Autodesk Inventor part; units mm, degrees
ref_plane "Work Plane1" through (104.775, 0, 0) normal (0, 0, -1) x (1, 0, 0)
ref_plane "YZ Plane" through (0, 0, 0) normal (1, 0, 0) x (0, 1, 0)
ref_plane "XZ Plane" through (0, 0, 0) normal (0, 1, 0) x (-1, 0, 0)
sketch "Esquisse1" plane through (0, 0, 0) normal (0, 0, 1) x (1, 0, 0)
  line L0 (16, 0) -> (16, 2)
  line L1 (16, 2) -> (4.6, 2)
  line L2 (4.6, 2) -> (4.1706, 2)
  line L3 (0, 4) -> (0, 1.4434)
  line L4 (0, 1.4434) -> (1.49, 1.4434)
  line L5 (1.49, 1.4434) -> (2.3233, 0)
  line L6 (2.3233, 0) -> (16, 0)
  line L7 (0, 4) -> (0.48, 4)
  line L8 (0.48, 4) -> (2.48, 2)
  line L9 (4.1706, 2) -> (2.48, 2)
  line L10 (4.6, 2) -> (2.48, 2) construction
  line L11 (2.48, 2) -> (2.48, 2)
  line L12 (-3.2, 0) -> (19.2, 0)
  line L13 (0, -0.8) -> (0, 4.8)
  dimension "d0" = 16
  dimension "d1" = 11.4
  dimension "d2" = 1.49
  dimension "d3" = 4
  dimension "d6" = 2.48
  dimension "d7" = 45
  dimension "d8" = 2.8868
  dimension "d9" = 60
  dimension "d10" = 8
  dimension "d11" = 4
  dimension "d12" = 0.4294
revolve "Corps" add sketch "Esquisse1" angle 360 about axis through (2.3233, 0, 0) along (1, 0, 0) contours L6 L5 L4 L3 L7 L8 L9 L2 L1 L0
sketch "Esquisse2" plane through (0, 0, 0) normal (-1, 0, 0) x (0, 0, 1)
  circle A0 centre (0, 0) radius 1.4434
  line L0 (0, -5.6) -> (0, 5.6)
  line L1 (-5.6, 0) -> (5.6, 0)
  line L2 (1.4434, 0) -> (0.7217, -1.25)
  line L3 (0.7217, -1.25) -> (-0.7217, -1.25)
  line L4 (-0.7217, -1.25) -> (-1.4434, 0)
  line L5 (-1.4434, 0) -> (-0.7217, 1.25)
  line L6 (-0.7217, 1.25) -> (0.7217, 1.25)
  line L7 (0.7217, 1.25) -> (1.4434, 0)
  point P0 (0, 1.4434)
extrude "Rainure" add sketch "Esquisse2" against normal up to next contours L7 A0 | A0 L2 | L6 L0 A0 | A0 L0 L3 | L0 L6 A0 | A0 L3 L0 | L4 A0 | A0 L5
thread "Filetage"
chamfer "Chanfrein1" distance 0.4294 distance2 0.4294 1 edges at (16, -2, 0) measured on face at (16, 0.2227, -0.5871)
ref_plane "Work Plane1" through (104.775, 0, 0) normal (0, 0, -1) x (1, 0, 0)
equation "\"d15\" = GEL"
equation "\"d17\" = -0.5 * SPD + 0.5 * GD"
equation "\"d18\" = GUL"
equation "\"d0\" = NLG"
equation "\"d1\" = GEL"
equation "\"d2\" = INTI"
equation "\"d3\" = GD"
equation "\"d6\" = KOH"
equation "\"d7\" = 0.5 * SEWI"
equation "\"d8\" = 1.1547 * SW"
equation "\"d10\" = KOD"
equation "\"d11\" = BDM"
equation "\"d12\" = GAL"
equation "\"NLG\" = 16"
equation "\"INTI\" = 1.49"
equation "\"GEL\" = 11.4"
equation "\"GAL\" = 0.61345 * PTC"
equation "\"KOH\" = 2.48"
equation "\"KOD\" = 8"
equation "\"GUL\" = 0.61345 * PTC"
equation "\"SPD\" = NND - 1.2269 * PTC"
equation "\"BDM\" = NND"
equation "\"GD\" = NND"
equation "\"SEWI\" = 90deg"
equation "\"SW\" = 2.5"
equation "\"TOA\" = 30deg"
equation "\"GD1\" = THREADDIA - 1.2269 * PTC"
equation "\"EPV\" = 4.48"
equation "\"THREADDIA\" = 4"
equation "\"PTC\" = 0.7"
equation "\"NND\" = 4"
equation "\"E0\" = 1.155 * SW"
properties part number "BS 4168 - M4 x 16" material "Acier, doux"
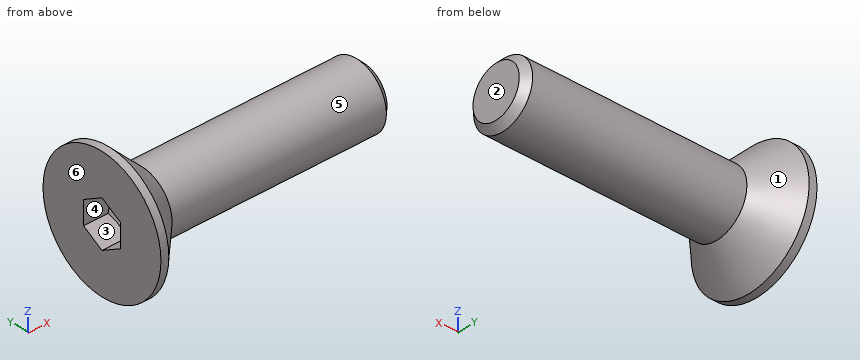
Geometry: final body of the model. Coordinates: model frame, mm. Face numbers are marked on the shaded views. A direction names the side the tool comes from. Round coordinates to 2 decimals unless told otherwise and drop trailing zeros. Write each loop counter-clockwise with the first axis right and the second up, starting at its lowest first coordinate (ties: lowest second). Pieces come first, ordered by that corner, then holes. Notation, with made-up numbers: (35.25, 87.25) -> (54.25, 87.25) arc R36 cw to (54.25, 121.25) -> close; hole circle Ø10 at (-39, -35.5). An arc over 180 degrees is marked (long way). Return JSON: item names as keys, results as strings.
Q1. Mould query, pull axis Z, two halves, no side actions, for the marked faces 1, 2 and 3. Classes: +Z half, -Z half, draft (parallel to the pull), parting line (faces both ways), or undercut.
From the geometry:
{"face 1": "parting line", "face 2": "draft", "face 3": "undercut"}
Q2. Set-up query: the marked faces 4, 5 and 6. Return all of +Z, -Z, +X, -X, +Y, -Y with unobstructed straight access to the full face (end or side cutting, diameter ignored); none if empty.
From the geometry:
{"face 4": "-X", "face 5": "+X", "face 6": "+Z, -Z, -X, +Y, -Y"}
Q3. Ray query, line 1 (X direction, y = -3.25, z = -0.25); line 2 (X direction, y = 1, z = 3.75); line 3 (Z direction, x = 10, y = -0.5). Return the intervals inside material, ascending.
From the geometry:
{"line 1": "0 to 1.22", "line 2": "0 to 0.6", "line 3": "-1.94 to 1.94"}
Q4. First-contact query: pin 1 Ø2 at (x, z) = (11, -1) entering from +Y; pin 2 Ø4 at (x, z) = (3, -1.5) entering from +Y; pin 3 Ø1 at (y, z) = (2, 0.5) entering from -X; pin 4 Ø2 at (x, y) = (5, 2.5) entering from +Z. Flat tips, straight axial feed; report the tip coordinate or a pass-through.
From the geometry:
{"pin 1": "y = 2", "pin 2": "y = 3.27", "pin 3": "x = 0", "pin 4": "z = 1.32"}
Q5. Section A-A on x = 1. Return the cut outline in (y, z), and give its area (3 significant figures).
From the geometry:
{"outline": "circle Ø6.96 at (0, 0); hole (-1.25, -0.72) -> (0, -1.44) -> (1.25, -0.72) -> (1.25, 0.72) -> (0, 1.44) -> (-1.25, 0.72) -> close", "area": "32.6 mm2"}
Q6. Section B-B on x = 3. Return the cut outline in (y, z).
From the geometry:
{"outline": "circle Ø4 at (0, 0)"}
